Work out the finished part from the listing and answer in its coordinate system (mm). Face numbers are marked on the shaded views. A direction names the side the tool comes from. Round coordinates to 2 decimals unless told otherwise and drop trailing zeros. Order: outer loops, then holes, each group sorted by start corner. A loop starts at its lowest first (then second) coordinate and runs counter-clockwise, first axis right, second up. Notation, with made-up numbers: (-36, 30) -> (-18, 30) arc R19 cw to (-18, 48) -> close; hole circle Ø6 at (-33.75, 9.5). An arc over 180 degrees is marked (long way). Use one line per item in the form item = value.
Autodesk Inventor part; units mm, degrees
ref_plane "YZ Plane" through (0, 0, 0) normal (1, 0, 0) x (0, 1, 0)
ref_plane "XZ Plane" through (0, 0, 0) normal (0, 1, 0) x (-1, 0, 0)
ref_plane "XY Plane" through (0, 0, 0) normal (0, 0, 1) x (1, 0, 0)
sketch "Sketch1" plane through (0, 0, 0) normal (0, 1, 0) x (-1, 0, 0)
  line L0 (-23.5, -19) -> (23.5, -19)
  line L1 (23.5, -19) -> (23.5, 19)
  line L2 (23.5, 19) -> (-23.5, 19)
  line L3 (-23.5, 19) -> (-23.5, -19)
  line L4 (-23.5, -19) -> (23.5, 19) construction
  line L5 (23.5, -19) -> (-23.5, 19) construction
  line L6 (-23, -18.5) -> (23, -18.5)
  line L7 (23, -18.5) -> (23, 18.5)
  line L8 (23, 18.5) -> (-23, 18.5)
  line L9 (-23, 18.5) -> (-23, -18.5)
  line L10 (-23, -18.5) -> (23, 18.5) construction
  line L11 (23, -18.5) -> (-23, 18.5) construction
  point P0 (0, 0)
  dimension "d0" = 47
  dimension "d1" = 38
  dimension "d2" = 46
  dimension "d3" = 37
extrude "Extrusion1" add sketch "Sketch1" along normal blind 2.5 contours L3 L2 L1 L0 | L9 L8 L7 L6
extrude "Extrusion2" add sketch "Sketch1" against normal blind 10
sketch "Sketch2" plane through (23.5, 2.5, 19) normal (1, 0, 0) x (0, 0, -1)
  line L0 (38, -12.5) -> (0, -12.5)
  line L1 (38, -12.5) -> (19, -12.5)
  line L2 (19, -12.5) -> (5, -12.5)
  point P0 (19, -2.5)
  dimension "d8" = 19
  dimension "d9" = 14
hole "Hole1" at (23.5, -10, 14) direction (-1, 0, 0) diameter 3.5 depth 8
hole "Hole2" at (23.5, -10, 0) direction (-1, 0, 0) diameter 11 depth 8
properties part number "HUDSON-1-54A"
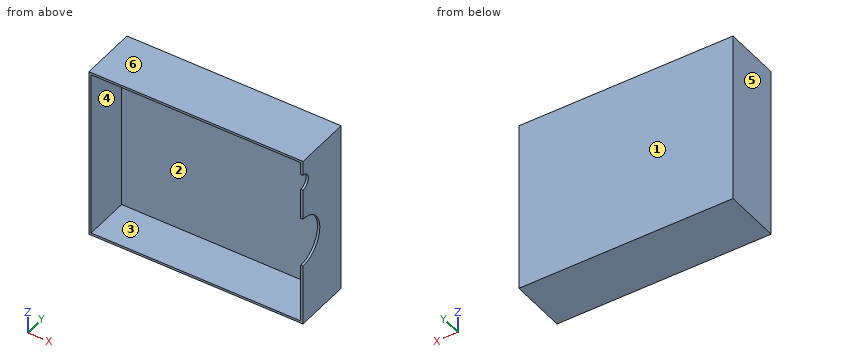
Item 1: The part is cut by section A-A, the plane y = -3. Give the vertices of the cut face in (x, z), and give its area (3 significant figures).
Findings:
outline = (-23.5, -19) -> (23.5, -19) -> (23.5, 19) -> (-23.5, 19) -> close; hole (-23, -18.5) -> (23, -18.5) -> (23, 18.5) -> (-23, 18.5) -> close
area = 84.0 mm^2
Item 2: The part is cut by section C-C, the plane y = -9. Give the vertices of the cut face in (x, z), and give its area (3 significant figures).
Findings:
outline = (-23.5, -19) -> (23.5, -19) -> (23.5, -5.41) -> (23, -5.41) -> (23, -18.5) -> (-23, -18.5) -> (-23, 18.5) -> (23, 18.5) -> (23, 15.44) -> (23.5, 15.44) -> (23.5, 19) -> (-23.5, 19) -> close; (23, 5.41) -> (23.5, 5.41) -> (23.5, 12.56) -> (23, 12.56) -> close
area = 77.2 mm^2
Item 3: For the marked faces 1 and 2, determine the directions among +Z, -Z, +X, -X, +Y, -Y from which every point of the face is accessible in a straight line to the end or side of a thin tool.
Findings:
face_1 = +Z, -Z, +X, -X, +Y
face_2 = -Y
Item 4: A flat-ended cylindrical pin translates along its axis: P1, Ø11, axis at x = -4.5, z = -4.5, coming from the -Y side. Find the tip coordinate at first contact, or state that the pin passes through.
Findings:
P1 = 0
Item 5: The part is cut by section D-D, the plane x = 0. Give the vertices of the cut face in (y, z), and give its area (3 significant figures).
Findings:
outline = (-10, -19) -> (2.5, -19) -> (2.5, 19) -> (-10, 19) -> (-10, 18.5) -> (0, 18.5) -> (0, -18.5) -> (-10, -18.5) -> close
area = 105 mm^2
Item 6: The part is cut by section B-B, the plane z = -13. Give the vertices of the cut face in (x, y).
Findings:
outline = (-23.5, -10) -> (-23, -10) -> (-23, 0) -> (23, 0) -> (23, -10) -> (23.5, -10) -> (23.5, 2.5) -> (-23.5, 2.5) -> close
Item 7: Consider line 1 along Z through (x, y) = (-19.5, -1.5); line 2 along X through (y, z) = (-0.75, 16); line 3 along Y through (x, z) = (11, 14.5). Determine where each line is inside the solid, lowest interval first.
Findings:
line_1 = -19 to -18.5, 18.5 to 19
line_2 = -23.5 to -23, 23 to 23.5
line_3 = 0 to 2.5
Item 8: Determine the mould class of the marked faces 3, 4, 5 and 6 for opening direction Z: released by +Z, released by -Z, zero draft, split by the parting line, or undercut.
Findings:
face_3 = undercut
face_4 = undercut
face_5 = zero draft
face_6 = released by +Z
